from build123d import *

# Parameters (mm, degrees)
SKETCH1_R           = 3.175
BOSS_EXTRUDE1_DEPTH = 210
BOSS_EXTRUDE2_START = -11.175
SKETCH2_R           = 2
BOSS_EXTRUDE2_DEPTH = 9.175


with BuildPart() as part:
    # Sketch1 → Boss-Extrude1 (new body)
    with BuildSketch(Plane.XY):
        Circle(SKETCH1_R)
    extrude(amount=BOSS_EXTRUDE1_DEPTH)

    # Sketch2 → Boss-Extrude2 (add)
    with BuildSketch(Plane(origin=(0, 0, 0), x_dir=(1, 0, 0), z_dir=(0, 1, 0)).offset(BOSS_EXTRUDE2_START)):
        with Locations(Location((0, -42.5, 0), (0, 0, 90))):
            Circle(SKETCH2_R)
        with Locations(Location((0, -190.5, 0), (0, 0, 90))):
            Circle(SKETCH2_R)
    extrude(amount=BOSS_EXTRUDE2_DEPTH)


solid = part.part
CAD build for the part. Positions are in the model's coordinates, mm. A direction names the side the tool comes from. Coordinates: 2 decimals unless noted, no trailing zeros. Order: outer loops, then holes, each group sorted by start corner. A loop starts at its lowest first (then second) coordinate and runs counter-clockwise, first axis right, second up.
Item 1: 3-axis set-ups, long thin cutter, end or side, ignore diameter. For faces 1 (the face through (0, 0, 210)), 2 (the face through (-0.088, -6.881, 44.498)): which of +Z, -Z, +X, -X, +Y, -Y reach the whole face in a straight line?
Check sheet entries:
face 1: +Z, +X, -X, +Y, -Y
face 2: -Y
Item 2: Two-plate mould, pull along Z, no slides. Class faces 3 (the face through (0, 0, 0)), 4 (the face through (-0.69, -3.1, 103.53)), 5 (the face through (0, -11.175, 191)): +Z half, -Z half, draft (parallel to the pull), parting line (faces both ways), or undercut.
Check sheet entries:
face 3: -Z half
face 4: undercut
face 5: draft
Item 3: Band-saw the part on D-D on z = 190.5. List the corners of the cut face in (x, y) (3 decimals), plus the area to 3 significant figures.
Check sheet entries:
outline: (-2, -11.175) - (2, -11.175) - (2, -2.466) arc R3.175 ccw (long way) to (-2, -2.466) - close
area: 64.6 mm2
Item 4: Drill centre lines: L1, parallel to Z at x = 0.25, y = -4; L2, parallel to Y at x = 0.25, z = 25.5; L3, parallel to Z at x = -0.5, y = -9. Where is each one in solid material? Low to high.
Check sheet entries:
L1: z = 40.52 to 44.48, 188.52 to 192.48
L2: y = -3.17 to 3.17
L3: z = 40.56 to 44.44, 188.56 to 192.44
Item 5: Band-saw the part on A-A on y = -9. List the corners of the cut face in (x, z).
Check sheet entries:
outline: circle Ø4 at (0, 42.5); circle Ø4 at (0, 190.5)
Item 6: Band-saw the part on C-C on z = 56. List the corners of the cut face in (x, y) (3 decimals).
Check sheet entries:
outline: circle Ø6.35 at (0, 0)
Item 7: Pin check, flat tips, straight feed: pin 1 Ø1.5 at (x, z) = (-2, 85.5) entering from +Y; pin 2 Ø2 at (x, y) = (1.5, -5) entering from -Z; pin 3 Ø1.5 at (x, z) = (2.5, 67) entering from -Y. Stop position of each tip, or through.
Check sheet entries:
pin 1: stops at y = 2.92
pin 2: stops at z = 40.56
pin 3: stops at y = -2.65
Item 8: Band-saw the part on B-B on x = 0. List the corners of the cut face in (y, z) (3 decimals), plus the area to 3 significant figures.
Check sheet entries:
outline: (-11.175, 40.5) - (-3.175, 40.5) - (-3.175, 0) - (3.175, 0) - (3.175, 210) - (-3.175, 210) - (-3.175, 192.5) - (-11.175, 192.5) - (-11.175, 188.5) - (-3.175, 188.5) - (-3.175, 44.5) - (-11.175, 44.5) - close
area: 1,400 mm2
